Part model, mm, in its own coordinate system. A direction names the side the tool comes from. Round coordinates to 2 decimals unless told otherwise and drop trailing zeros. Loops run counter-clockwise (first coordinate to the right, second up) from the corner with the lowest first, then second, coordinate; pieces in that order, holes last. Notation, with made-up numbers: (36, 79.25) - (51, 79.25) arc R27 cw to (51, 97.25) - close; hole circle Ø7 at (51, 67.5). An arc over 180 degrees is marked (long way). Write each question's results on one line, items separated by ' | '. Start each with the question number.
(1) Cut at D-D, the plane y = -1.85. List the corners of the cut face in (x, z).
(2) Cut at C-C, the plane z = 7.5. List the corners of the cut face in (x, y), then the cut area to 3 significant figures.
(3) Drill centre lines: L1, parallel to Y at x = 0, z = 3.05; L2, parallel to Z at x = 2.1, y = 0.5; L3, parallel to Z at x = 0.35, y = -0.9. Where is each one in solid material? Low to high.
(4) Cut at B-B, the plane z = 1.75. List the corners of the cut face in (x, y), then the cut area to 3 significant figures.
(5) Tool access for faces 1 (the face through (0, 2, 0)), 2 (the face through (0, 2, 11)), 3 (the face through (0, 0, 6)): list every direction of +Z, -Z, +X, -X, +Y, -Y with a clear straight run to the whole face (end or side of a thin tool).
(6) Cut at A-A, the plane x = 0. List the corners of the cut face in (y, z).
(7) Mould opens along X. For faces 4 (the face through (2.001, -1.134, 5.423)), 5 (the face through (-2.001, 1.134, 5.423)), 6 (the face through (1.5, 0.07, 2.96)) say: released by +X, released by -X, zero draft, split by the parting line, or undercut.
(8) Flat gauge pins, fed straight in: P1, Ø1.5, axis at x = -2, y = 1.5, coming from the -Z side; P2, Ø1.5, axis at x = -2, z = 15, coming from the +Y side; P3, Ø1.5, axis at y = 2, z = 6, coming from the +X side. Where does each tip first touch, or does it go through?
Autodesk Inventor part; units mm, degrees
ref_plane "YZ Plane" through (0, 0, 0) normal (1, 0, 0) x (0, 1, 0)
ref_plane "XZ Plane" through (0, 0, 0) normal (0, 1, 0) x (-1, 0, 0)
ref_plane "XY Plane" through (0, 0, 0) normal (0, 0, 1) x (1, 0, 0)
sketch "Base" plane through (0, 0, 0) normal (0, 0, 1) x (1, 0, 0)
  line L0 (1.3279, 2.3) -> (2.6558, 0)
  line L1 (2.6558, 0) -> (1.3279, -2.3)
  line L2 (1.3279, -2.3) -> (-1.3279, -2.3)
  line L3 (-1.3279, -2.3) -> (-2.6558, 0)
  line L4 (-2.6558, 0) -> (-1.3279, 2.3)
  line L5 (-1.3279, 2.3) -> (1.3279, 2.3)
  line L6 (-3.7181, 0) -> (3.7181, 0) construction
  line L7 (0, -3.22) -> (0, 3.22) construction
  point P0 (0, 0)
  point P1 (0, 0)
  dimension "d0" = 4.6
extrude "BaseFeature" add sketch "Base" along normal blind 11
sketch "Sketch2" plane through (0, 0, 11) normal (0, 0, 1) x (1, 0, 0)
  circle A0 centre (0, 0) radius 1.5
  dimension "d3" = 3
extrude "Extrusion2" add sketch "Sketch2" along normal blind 6
chamfer "Chamfer1" distance 0.5 angle 45 1 edges at (-1.5, 0, 17)
sketch "Sketch3" plane through (0, 0, 0) normal (0, 0, -1) x (-1, 0, 0)
  circle A0 centre (0, 0) radius 1.5
  dimension "d9" = 3
extrude "Extrusion3" cut sketch "Sketch3" against normal blind 6
properties part number "UXCell-M3x11-MaleFemaleHexStandoff"
A:
1) outline: (-1.59, 0) - (1.59, 0) - (1.59, 11) - (-1.59, 11) - close
2) outline: (-2.66, 0) - (-1.33, -2.3) - (1.33, -2.3) - (2.66, 0) - (1.33, 2.3) - (-1.33, 2.3) - close | area: 18.3 mm2
3) L1: -2.3 to -1.5, 1.5 to 2.3 | L2: 0 to 11 | L3: 6 to 17
4) outline: (-2.66, 0) - (-1.33, -2.3) - (1.33, -2.3) - (2.66, 0) - (1.33, 2.3) - (-1.33, 2.3) - close; hole circle Ø3 at (0, 0) | area: 11.3 mm2
5) face 1: -Z, +X, -X, +Y, -Y | face 2: +Z | face 3: -Z
6) outline: (-2.3, 0) - (-1.5, 0) - (-1.5, 6) - (1.5, 6) - (1.5, 0) - (2.3, 0) - (2.3, 11) - (1.5, 11) - (1.5, 16.5) - (1, 17) - (-1, 17) - (-1.5, 16.5) - (-1.5, 11) - (-2.3, 11) - close
7) face 4: released by +X | face 5: released by -X | face 6: undercut
8) P1: z = 0 | P2: y = 0.83 | P3: x = 1.93
